from build123d import *

# Parameters (mm, degrees)
F1_DEPTH       = 50.8
F3_D           = 13.49248
F3_CSINK_D     = 23.8252
F3_CSINK_ANGLE = 82
F4_R           = 6.35
F5_SIZE        = 0.8128
F7_D           = 25.4


with BuildPart() as f1:
    # F0 (on Front) → F1 (new body, symmetric)
    with BuildSketch(Plane.XZ):
        Polygon((-6.35, 25.4), (-50.8, 25.4), (-50.8, -25.4), (50.8, -25.4), (50.8, 25.4), (6.35, 25.4), (6.35, 19.05), (0, 19.05), (-6.35, 19.05), align=None)
    extrude(amount=F1_DEPTH, both=True)

    # F3 (through all)
    with Locations(Plane.XY.offset(25.4)):
        with Locations((-31.75, 31.75), (31.75, 31.75), (-31.75, -31.75), (31.75, -31.75)):
            CounterSinkHole(F3_D / 2, F3_CSINK_D / 2, counter_sink_angle=F3_CSINK_ANGLE)

    # F4
    f4_edges = [f1.edges().sort_by_distance(p)[0] for p in [
        (-50.8, 50.8, 0),
        (-50.8, -50.8, 0),
        (50.8, -50.8, 0),
        (50.8, 50.8, 0),
    ]]
    fillet(f4_edges, radius=F4_R)

    # F5
    f5_edges = [f1.edges().sort_by_distance(p)[0] for p in [
        (50.8, 0, 25.4),
        (-25.4, 50.8, 25.4),
        (25.4, 50.8, 25.4),
        (-50.8, 0, 25.4),
        (-25.4, -50.8, 25.4),
        (25.4, -50.8, 25.4),
        (-50.8, 0, -25.4),
        (-48.940128, 48.940128, -25.4),
        (-48.940128, -48.940128, -25.4),
        (0, 50.8, -25.4),
        (0, -50.8, -25.4),
        (48.940128, 48.940128, -25.4),
        (48.940128, -48.940128, -25.4),
        (50.8, 0, -25.4),
        (-38.49624, 31.75, -25.4),
        (25.00376, 31.75, -25.4),
        (-38.49624, -31.75, -25.4),
        (25.00376, -31.75, -25.4),
    ]]
    chamfer(f5_edges, length=F5_SIZE)

    # F7 (through all)
    with Locations(Plane.XZ.offset(50.8)):
        with Locations((0, 0)):
            Hole(F7_D / 2)


solid = f1.part
Verification items for the finished model (mm, model axes). A direction names the side the tool comes from. Round coordinates to 2 decimals unless told otherwise and drop trailing zeros. Order: outer loops, then holes, each group sorted by start corner. A loop starts at its lowest first (then second) coordinate and runs counter-clockwise, first axis right, second up.
1. Thickness scan on L1, parallel to Y at x = -31.75, z = -8.5; L2, parallel to Z at x = 0, y = 2.5; L3, parallel to Z at x = 11, y = 24. Record the ranges inside material, lowest first.
Final values:
L1: y = -50.8 to -38.5, -25 to 25, 38.5 to 50.8
L2: z = -25.4 to -12.7, 12.7 to 19.05
L3: z = -25.4 to -6.35, 6.35 to 25.4
2. Section check B-B on x = 0. Record the cut outline in (y, z).
Final values:
outline: (-50.8, -24.59) - (-49.99, -25.4) - (49.99, -25.4) - (50.8, -24.59) - (50.8, -12.7) - (-50.8, -12.7) - close; (-50.8, 12.7) - (50.8, 12.7) - (50.8, 19.05) - (-50.8, 19.05) - close
3. Release check for a two-part mould opening along X. For faces 1 (the conical face through (48.42, 48.51, 25.26)), 2 (the flat face through (-1, -1, -25.4)), 3 (the conical face through (37.303, -36.008, 19.745)) record: +X half, -X half, draft (parallel to the pull), parting line (faces both ways), or undercut.
Final values:
face 1: +X half
face 2: draft
face 3: undercut
4. Go/stop test with flat-tipped pins: P1, Ø4, axis at x = 1, y = 19.5, coming from the +Z side; P2, Ø4, axis at x = -38, y = 30.5, coming from the +Z side. Record where each tip stops, or that it passes through.
Final values:
P1: stops at z = 19.05
P2: stops at z = 21.33
5. Section check D-D on x = 31.75. Record the cut outline in (y, z).
Final values:
outline: (-50.8, -24.59) - (-49.99, -25.4) - (-39.31, -25.4) - (-38.5, -24.59) - (-38.5, 19.46) - (-43.66, 25.4) - (-49.99, 25.4) - (-50.8, 24.59) - close; (-25, -24.59) - (-24.19, -25.4) - (24.19, -25.4) - (25, -24.59) - (25, 19.46) - (19.84, 25.4) - (-19.84, 25.4) - (-25, 19.46) - close; (38.5, -24.59) - (39.31, -25.4) - (49.99, -25.4) - (50.8, -24.59) - (50.8, 24.59) - (49.99, 25.4) - (43.66, 25.4) - (38.5, 19.46) - close
6. Section check A-A on z = 0. Record the cut outline in (x, y), then the cut area to 3 significant figures.
Final values:
outline: (-50.8, -44.45) arc R6.35 ccw to (-44.45, -50.8) - (-12.7, -50.8) - (-12.7, 50.8) - (-44.45, 50.8) arc R6.35 ccw to (-50.8, 44.45) - close; (12.7, -50.8) - (44.45, -50.8) arc R6.35 ccw to (50.8, -44.45) - (50.8, 44.45) arc R6.35 ccw to (44.45, 50.8) - (12.7, 50.8) - close; hole circle Ø13.49 at (-31.75, -31.75); hole circle Ø13.49 at (-31.75, 31.75); hole circle Ø13.49 at (31.75, -31.75); hole circle Ø13.49 at (31.75, 31.75)
area: 7,140 mm2
7. Section check C-C on z = -17. Record the cut outline in (x, y), then the cut area to 3 significant figures.
Final values:
outline: (-50.8, -44.45) arc R6.35 ccw to (-44.45, -50.8) - (44.45, -50.8) arc R6.35 ccw to (50.8, -44.45) - (50.8, 44.45) arc R6.35 ccw to (44.45, 50.8) - (-44.45, 50.8) arc R6.35 ccw to (-50.8, 44.45) - close; hole circle Ø13.49 at (-31.75, -31.75); hole circle Ø13.49 at (-31.75, 31.75); hole circle Ø13.49 at (31.75, -31.75); hole circle Ø13.49 at (31.75, 31.75)
area: 9,720 mm2
8. Access from +Z, -Z, +X, -X, +Y, -Y to the whole of each face (thin tool, end or side, straight path). Record for faces 4 (the flat face through (-6.35, -1, 22)), 5 (the conical face through (-48.42, 48.51, 25.26)).
Final values:
face 4: +Z, +Y, -Y
face 5: +Z, -X, +Y
